Autodesk Inventor part; units mm, degrees
ref_plane "YZ Plane" through (0, 0, 0) normal (1, 0, 0) x (0, 1, 0)
ref_plane "XZ Plane" through (0, 0, 0) normal (0, 1, 0) x (-1, 0, 0)
ref_plane "XY Plane" through (0, 0, 0) normal (0, 0, 1) x (1, 0, 0)
sketch "Sketch1" plane through (0, 0, 0) normal (1, 0, 0) x (0, 1, 0)
  line L0 (-25.4, -22.225) -> (0, -22.225)
  line L1 (0, -22.225) -> (0, 22.225) construction
  line L2 (0, 22.225) -> (-25.4, 22.225)
  line L3 (-25.4, 22.225) -> (-25.4, -22.225) construction
  line L4 (-25.4, 0) -> (0, 0) construction
  arc A0 (0, -22.225) -> (0, 22.225) centre (0, 0) ccw
  circle A1 centre (-25.4, 0) radius 3.81 construction
  circle A2 centre (0, 0) radius 3.81
  line L5 (-25.4, 22.225) -> (-38.1, 22.225)
  line L6 (-38.1, 22.225) -> (-38.1, -22.225)
  line L7 (-38.1, -22.225) -> (-25.4, -22.225)
  line L8 (0, -5.7) -> (0, 5.7) construction
  line L9 (5.6896, 0) -> (-18.1104, 0) construction
  point P0 (0, 0)
  dimension "d0" = 25.4
  dimension "d1" = 44.45
  dimension "d2" = 7.62
  dimension "d3" = 12.7
extrude "Extrusion1" add sketch "Sketch1" along normal blind 5.08 contours L7 L6 L5 L2 A0 L0 | A2
sketch "Sketch2" plane through (0, 0, 0) normal (-1, 0, 0) x (0, 0, 1)
  line L0 (-22.225, -38.1) -> (-22.225, 0)
  line L1 (22.225, -38.1) -> (-22.225, -38.1)
  line L2 (22.225, 0) -> (22.225, -38.1)
  line L3 (-22.225, 0) -> (22.225, 0) construction
  line L4 (-22.225, -12.7) -> (-17.145, -12.7)
  line L5 (-17.145, -12.7) -> (-17.145, -31.75)
  line L6 (-17.145, -31.75) -> (-22.225, -31.75)
  line L7 (-22.225, -31.75) -> (-22.225, -12.7)
  line L8 (22.225, -12.7) -> (17.145, -12.7)
  line L9 (17.145, -12.7) -> (17.145, -31.75)
  line L10 (17.145, -31.75) -> (22.225, -31.75)
  line L11 (22.225, -31.75) -> (22.225, -12.7)
  line L12 (0, -38.1) -> (0, 0)
  dimension "d12" = 38.1
  dimension "d13" = 5.08
  dimension "d14" = 5.08
  dimension "d15" = 19.05
  dimension "d16" = 12.7
extrude "Extrusion2" cut sketch "Sketch2" against normal through all
sketch "Sketch3" plane through (0, 0, 0) normal (-1, 0, 0) x (0, 0, 1)
  arc A0 (22.225, 0) -> (-22.225, 0) centre (0, 0) ccw
  circle A1 centre (0, 0) radius 6.35
  dimension "d19" = 12.7
extrude "Extrusion3" add sketch "Sketch3" along normal blind 2.54
sketch "Sketch4" plane through (-2.54, 0, 0) normal (-1, 0, 0) x (0, 0, 1)
  circle A0 centre (0, 0) radius 6.35
  circle A1 centre (0, 0) radius 3.81
  dimension "d22" = 7.62
extrude "Extrusion4" add sketch "Sketch4" along normal blind 5.08 contours A1
sketch "Sketch5" plane through (-7.62, 0, 0) normal (-1, 0, 0) x (0, 0, 1)
  circle A0 centre (0, 0) radius 3.81
  line L0 (-3.81, 0) -> (3.81, 0)
revolve "Revolution1" add sketch "Sketch5" angle 180 about axis through (-7.62, 0, -3.81) along (0, 0, 1) picked at (0.9506, 0.8422) contours L0 A0
sketch "Sketch6" plane through (0, 0, 0) normal (-1, 0, 0) x (0, 0, 1)
  line L0 (-22.225, -38.1) -> (-22.225, -31.75)
  line L1 (22.225, -38.1) -> (-22.225, -38.1)
  line L2 (-22.225, -12.7) -> (-17.145, -12.7)
  line L3 (-17.145, -12.7) -> (-17.145, -31.75)
  line L4 (-22.225, -31.75) -> (-23.8687, -31.75)
  spline S0 degree 3 poles (-24.3389, -38.1) (-24.1438, -35.6808) (-23.9932, -34.219) (-23.8687, -31.75) knots -0.835253 -0.835253 -0.835253 -0.835253 -0.05147 -0.05147 -0.05147 -0.05147
  line L5 (-22.225, -38.1) -> (-24.3389, -38.1)
  line L6 (-17.145, -38.1) -> (-17.145, -31.75)
  line L7 (-23.3095, -12.7) -> (-22.225, -12.7)
  line L8 (-17.145, -12.7) -> (-17.145, 0)
  line L9 (-17.145, 0) -> (-22.225, 0)
  spline S1 degree 3 poles (-23.3095, -12.7) (-23.2316, -10.9447) (-23.0986, -8.2586) (-22.7786, -3.8937) (-22.5606, -1.8124) (-22.225, 0) knots -1.036051 -1.036051 -1.036051 -1.036051 -0.552963 -0.552963 0 0 0 0
  line L10 (-22.225, -12.7) -> (-22.225, 0)
  line L11 (-22.225, -31.75) -> (-22.225, -38.1)
  dimension "d26" = 6.35
  dimension "d27" = 6.7237
  dimension "d28" = 7.1939
  dimension "d29" = 12.7
  dimension "d30" = 6.1645
  dimension "d31" = 5.08
extrude "Extrusion5" add sketch "Sketch6" against normal up to surface (5.08 mm away) contours L5 S0 L4 L0 | L7 S1 L10
sketch "Sketch7" plane through (0, -12.7, -17.145) normal (0, -1, 0) x (1, 0, 0)
  line L0 (0, 0) -> (5.08, 0)
  line L1 (0, -6.1645) -> (5.08, -6.1645)
  line L2 (10.233, 22.3578) -> (10.233, -6.8582) construction
  line L3 (5.08, 0) -> (0, 0)
  line L4 (5.08, -6.1645) -> (5.08, 0)
  spline S0 degree 3 poles (0, -5.08) (1.6825, -5.4909) (3.3765, -5.8525) (5.08, -6.1645) knots -0.570375 -0.570375 -0.570375 -0.570375 -0.050806 -0.050806 -0.050806 -0.050806
  line L5 (0, -5.08) -> (0, 0)
  line L6 (0, 39.37) -> (0, -7.1939)
  line L7 (0, -5.08) -> (0, -6.1645)
  line L8 (5.08, -6.1645) -> (0, -6.1645)
  point P0 (0, 17.145)
  dimension "d37" = 5.08
  dimension "d38" = 6.1645
  dimension "d39" = 5.08
extrude "Extrusion6" cut sketch "Sketch7" against normal through all contours S0 L1 L6
sketch "Sketch8" plane through (0, -31.75, -17.145) normal (0, 1, 0) x (1, 0, 0)
  line L0 (0, 0) -> (5.08, 0)
  line L1 (0, 5.08) -> (0, 0)
  spline S0 degree 3 poles (5.08, 6.7237) (3.3633, 6.251) (1.6683, 5.7026) (0, 5.08) knots -0.534217 -0.534217 -0.534217 -0.534217 0 0 0 0
  line L2 (5.08, 0) -> (5.08, 6.7237)
  line L3 (5.08, 6.1645) -> (5.08, 0)
  line L4 (0, 0) -> (5.08, 0)
  line L5 (5.08, 6.7237) -> (0, 6.7237)
  line L6 (0, 6.7237) -> (0, 5.08)
  line L7 (5.08, 6.7237) -> (5.08, 7.1939)
  line L8 (0, 7.1939) -> (5.08, 7.1939)
  line L9 (0, 6.7237) -> (0, 7.1939)
  line L10 (0, 6.7237) -> (5.08, 6.7237)
  line L11 (0, 6.7237) -> (5.08, 6.7237)
  line L12 (5.08, 6.7237) -> (5.08, 7.1939)
  line L13 (5.08, 7.1939) -> (0, 7.1939)
  line L14 (0, 7.1939) -> (0, 6.7237)
  point P0 (0, -17.145)
  dimension "d42" = 5.08
  dimension "d43" = 5.08
  dimension "d44" = 6.7237
extrude "Extrusion7" cut sketch "Sketch8" against normal through all contours L6 L5 S0 | L5 L9 L8 L7
sketch "Sketch9" plane through (0, 0, 0) normal (-1, 0, 0) x (0, 0, 1)
  line L0 (22.225, -38.1) -> (-22.225, -38.1)
  line L1 (-17.145, -31.75) -> (-22.225, -31.75)
  line L2 (-17.145, -31.75) -> (-17.145, -38.1) construction
  line L3 (17.145, -31.75) -> (17.145, -38.1) construction
  arc A0 (17.145, -38.1) -> (-17.145, -38.1) centre (0, -50.1877) ccw
  line L4 (0, -38.1) -> (0, -29.21) construction
  dimension "d47" = 8.89
extrude "Extrusion8" cut sketch "Sketch9" against normal through all
fillet "Fillet1" radius 2.54 2 edges at (0, 0, -6.35) (-2.54, 0, -6.35)
properties part number "upper_pin"
The model under review builds one solid part; all positions refer to its coordinate system, in mm. A direction names the side the tool comes from. Round coordinates to 2 decimals unless told otherwise and drop trailing zeros. Loops run counter-clockwise (first coordinate to the right, second up) from the corner with the lowest first, then second, coordinate; pieces in that order, holes last.
Item 1: For line 1 (X direction, y = -11.5, z = -20); line 2 (Y direction, x = 3, z = -20.5); line 3 (Y direction, x = 4, z = -10), list the stretches that pass through material, from the lowest coordinate up.
Determined:
line 1: x = 0 to 5.08
line 2: y = -38.1 to -31.75, -12.7 to 8.58
line 3: y = -31.75 to 19.85
Item 2: Take a section at A-A (z = 18). Write out the cut boundary in (x, y).
Determined:
outline: (0, -38.1) - (5.08, -38.1) - (5.08, -31.75) - (0, -31.75) - close; (0, -12.7) - (5.08, -12.7) - (5.08, 13.04) - (0, 13.04) - close
Item 3: Take a section at D-D (z = -20). Write out the cut boundary in (x, y).
Determined:
outline: (0, -38.1) - (5.08, -38.1) - (5.08, -31.75) - (0, -31.75) - close; (0, -12.7) - (5.08, -12.7) - (5.08, 9.69) - (0, 9.69) - close
Item 4: Mouldability with a two-part tool opening along Y and no side actions: class faces 1 (the face through (3, -22, 17.145)), 2 (the face through (3, -6, 22.225)), 3 (the face through (2.5, 22.22, 0.49)), 4 (the face through (3, -22, -17.145)) as released by +Y, released by -Y, zero draft, split by the parting line, or undercut.
Determined:
face 1: undercut
face 2: zero draft
face 3: released by +Y
face 4: undercut
Item 5: Take a section at B-B (x = -5.25). Write out the cut boundary in (y, z), then the cut area to 3 significant figures.
Determined:
outline: circle Ø7.62 at (0, 0)
area: 45.6 mm2
Item 6: Take a section at C-C (y = -27.5). Write out the cut boundary in (x, z) (3 decimals).
Determined:
outline: (0, -17.145) - (5.08, -17.145) - (5.08, 17.145) - (0, 17.145) - close
Item 7: For faces 5 (the face through (2.5, -29.21, 0.28)), 6 (the face through (-5.04, 3.72, -0.83)), 7 (the face through (3, -12.7, 20)), list the 3-axis set-ups (+Z, -Z, +X, -X, +Y, -Y) from which the entire face can be reached by the end or side of a thin tool; tool diameter is ignored.
Determined:
face 5: +X, -X, -Y
face 6: -X
face 7: +Z, +X, -X
Item 8: Clearance check with flat-ended pins moving along their axes: pin 1 Ø2.5 at (y, z) = (2, 2) entering from -X; pin 2 Ø5.5 at (x, z) = (1.5, -18.5) entering from +Y; pin 3 Ø6 at (y, z) = (12, 9.5) entering from -X. State where each tip first meets the part, or that it passes through.
Determined:
pin 1: stops at x = -11.09
pin 2: stops at y = 15.68
pin 3: stops at x = 0
